Could you check a few things on this model? Use its own coordinates, in mm. Face numbers are marked on the shaded views. A direction names the side the tool comes from. Give positions to 0.01 mm unless a question says otherwise; leave off trailing zeros. Loops run counter-clockwise (first coordinate to the right, second up) from the corner with the lowest first, then second, coordinate; pieces in that order, holes last. Notation, with made-up numbers: M 25.5,9.25 L 64.5,9.25 A23 cw 64.5,37.25 Z; hole C -12,12 d3. An arc over 180 degrees is marked long. Use a Markdown table: item, result. Add a question column.
1) Suppose I cut it at C-C on x = -32.5. List the corners of the cut face in (y, z) for me.
2) Which directions (+Z, -Z, +X, -X, +Y, -Y) give clear straight access to the entire face, cutting with the end or side of a thin tool? Please do the marked faces 1, 2 and 3.
3) If I drill on line 1 along Y through (x, z) = (-34, 7); line 2 along Z through (x, y) = (-22.5, -11); line 3 along Z through (x, y) = (-11, 13.5), over which ranges is the centre line in solid material (lowest first)? Write a range as [from, to].
4) Will these pins go through, and if not, where does the flat tip stop? pin 1 Ø3 at (x, y) = (-22, 2) entering from +Z; pin 2 Ø1.1 at (x, z) = (-7.5, -0.5) entering from -Y; pin 3 Ø12 at (x, z) = (-22, 45.5) entering from -Y.
5) Suppose I cut it at B-B on z = 29. List the corners of the cut face in (x, y) for me.
6) Suppose I cut it at D-D on y = 7. List the corners of the cut face in (x, z) for me.
7) Suppose I cut it at A-A on x = -11. List the corners of the cut face in (y, z) for me, and give its area (3 significant figures).
```python
from build123d import *

# Parameters (mm, degrees)
BASE_FLANGE1_DEPTH           = 1
EDGE_FLANGE1_STRIP_W         = 7.2
EDGE_FLANGE1_STRIP_H         = 1
EDGE_FLANGE1_STRIP_CUT_DEPTH = 40
EDGE_FLANGE1_DEPTH           = 40
EDGE_FLANGE2_STRIP_W         = 7.2
EDGE_FLANGE2_STRIP_H         = 1
EDGE_FLANGE2_STRIP_CUT_DEPTH = 40
EDGE_FLANGE2_DEPTH           = 40


# Sheet-metal steps are written as plain solids
with BuildPart() as part:
    # Sketch1 → Base-Flange1 (new body)
    with BuildSketch(Plane.XY):
        Polygon((0, 0), (0, 3), (-40, 3), (-40, -52), (-18.16511543, -52), (-17.7, 0), align=None)
    extrude(amount=-BASE_FLANGE1_DEPTH)

    # Edge-Flange1 strip (across the edge) → Edge-Flange1 strip cut (cut)
    with BuildSketch(Plane(origin=(0, 3, 0), x_dir=(0, -1, 0), z_dir=(-1, 0, 0))):
        with Locations((-1, -0.5)):
            Rectangle(EDGE_FLANGE1_STRIP_W, EDGE_FLANGE1_STRIP_H)
    extrude(amount=EDGE_FLANGE1_STRIP_CUT_DEPTH, mode=Mode.SUBTRACT)

    # Edge-Flange1 section (across the edge) → Edge-Flange1 (add)
    with BuildSketch(Plane(origin=(0, 3, 0), x_dir=(0, -1, 0), z_dir=(-1, 0, 0))):
        with BuildLine():
            Line((0, 1.6), (0, 63))
            Line((0, 63), (1, 63))
            Line((1, 63), (1, 1.6))
            ThreePointArc((1, 1.6), (1.46862915, 0.46862915), (2.6, 0))
            Line((2.6, 0), (2.6, -1))
            ThreePointArc((2.6, -1), (0.761522369, -0.238477631), (0, 1.6))
        make_face()
    extrude(amount=EDGE_FLANGE1_DEPTH)

    # Edge-Flange2 strip (across the edge) → Edge-Flange2 strip cut (cut)
    with BuildSketch(Plane(origin=(-40, 3, 63), x_dir=(0, 0, -1), z_dir=(1, 0, 0))):
        with Locations((-1, -0.5)):
            Rectangle(EDGE_FLANGE2_STRIP_W, EDGE_FLANGE2_STRIP_H)
    extrude(amount=EDGE_FLANGE2_STRIP_CUT_DEPTH, mode=Mode.SUBTRACT)

    # Edge-Flange2 section (across the edge) → Edge-Flange2 (add)
    with BuildSketch(Plane(origin=(-40, 3, 63), x_dir=(0, 0, -1), z_dir=(1, 0, 0))):
        with BuildLine():
            Line((0, 1.6), (0, 13))
            Line((0, 13), (1, 13))
            Line((1, 13), (1, 1.6))
            ThreePointArc((1, 1.6), (1.46862915, 0.46862915), (2.6, 0))
            Line((2.6, 0), (2.6, -1))
            ThreePointArc((2.6, -1), (0.761522369, -0.238477631), (0, 1.6))
        make_face()
    extrude(amount=EDGE_FLANGE2_DEPTH)


solid = part.part
```
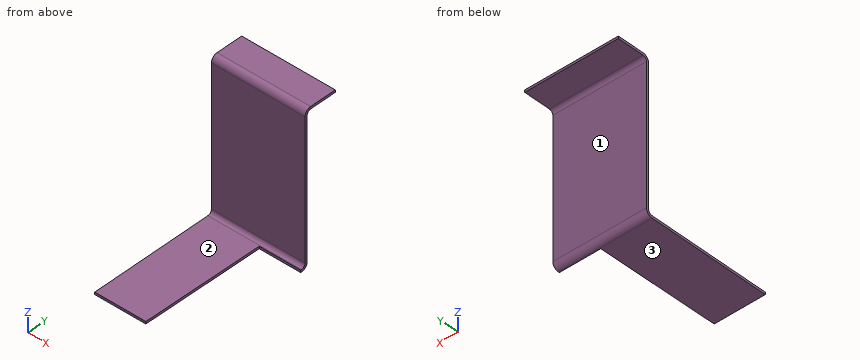
Answer block:
| question | item | result |
|---|---|---|
| 1 | outline | M -52,-1 L 0.4,-1 A2.6 ccw 3,1.6 L 3,60.4 A1.6 cw 4.6,62 L 16,62 L 16,63 L 4.6,63 A2.6 ccw 2,60.4 L 2,1.6 A1.6 cw 0.4,0 L -52,0 Z |
| 2 | face 1 | -Z, +X, -X, +Y |
| 2 | face 2 | +Z, +X, -X, -Y |
| 2 | face 3 | -Z, +X, -X, +Y, -Y |
| 3 | line 1 | y = [2, 3] |
| 3 | line 2 | z = [-1, 0] |
| 3 | line 3 | z = [62, 63] |
| 4 | pin 1 | stops at z = 62.76 |
| 4 | pin 2 | stops at y = 0 |
| 4 | pin 3 | stops at y = 2 |
| 5 | outline | M -40,2 L 0,2 L 0,3 L -40,3 Z |
| 6 | outline | M -40,62 L 0,62 L 0,63 L -40,63 Z |
| 7 | outline | M 0,-1 L 0.4,-1 A2.6 ccw 3,1.6 L 3,60.4 A1.6 cw 4.6,62 L 16,62 L 16,63 L 4.6,63 A2.6 ccw 2,60.4 L 2,1.6 A1.6 cw 0.4,0 L 0,0 Z |
| 7 | area | 77.2 mm^2 |
